Geometry check sheet. Reference: the model listing, model coordinates, mm. Give positions to 0.01 mm unless a question says otherwise; leave off trailing zeros. Order: outer loops, then holes, each group sorted by start corner. A loop starts at its lowest first (then second) coordinate and runs counter-clockwise, first axis right, second up. Notation, with made-up numbers: M 56.25,-34.5 L 88.25,-34.5 A31 ccw 88.25,-8.5 Z; hole C 69.25,71 d1. An arc over 180 degrees is marked long. Put each result on its own line as item: value. Start each with the question number.
Q1. Go/stop test with a flat-tipped pin: pin 1 (5.5 mm diameter, centred on x = -36, z = -4, fed in from -Y). Record where the tip stops, or that it passes through.
Q2. Section check C-C on y = 191. Record the cut outline in (x, z) (3 decimals), then the cut area to 3 significant figures.
Q3. Section check B-B on x = -40.5. Record the cut outline in (y, z) (3 decimals), then the cut area to 3 significant figures.
Q4. Section check D-D on z = -4.5. State how many separate pieces and enclosed holes the cut face has, then the cut area to 3 significant figures.
Q5. Material ranges on L1, parallel to X at y = -75.5, z = -6; L2, parallel to X at y = 268.5, z = 7.5; L3, parallel to Y at x = 256.5, z = -2, recorded low to high.
Q6. Section check A-A on x = 291. Record the cut outline in (y, z) (3 decimals).
```python
from build123d import *

# Parameters (mm, degrees)
SKETCH1_W           = 914.4
SKETCH1_H           = 914.4
BOSS_EXTRUDE1_DEPTH = 9.525
SKETCH2_W           = 184
SKETCH2_H           = 285
SKETCH2_W_2         = 300
SKETCH2_H_2         = 495
SKETCH2_W_3         = 469.9
SKETCH2_H_3         = 685.8
SKETCH2_H_4         = 177.8
CUT_EXTRUDE1_DEPTH  = 647.859012846
FILLET1_R           = 1


with BuildPart() as part:
    # Sketch1 → Boss-Extrude1 (new, symmetric)
    with BuildSketch(Plane.XY):
        Rectangle(SKETCH1_W, SKETCH1_H)
    extrude(amount=BOSS_EXTRUDE1_DEPTH, both=True)

    # Sketch2 → Cut-Extrude1 (cut, through all)
    with BuildSketch(Plane.XY.offset(9.525)):
        with Locations((292.1, 254)):
            Rectangle(SKETCH2_W, SKETCH2_H)
        with Locations((292.1, -177.8)):
            Rectangle(SKETCH2_W_2, SKETCH2_H_2)
        with Locations((-125.73, 101.6)):
            Rectangle(SKETCH2_W_3, SKETCH2_H_3)
        with Locations((-125.73, -368.3)):
            Rectangle(SKETCH2_W_3, SKETCH2_H_4)
    extrude(amount=-CUT_EXTRUDE1_DEPTH, mode=Mode.SUBTRACT)

    # Fillet1
    fillet1_edges = [part.edges().sort_by_distance(p)[0] for p in [
        (142.1, -425.3, 0),
        (142.1, 69.7, 0),
        (442.1, 69.7, 0),
        (442.1, -425.3, 0),
        (-360.68, -241.3, 0),
        (-360.68, 444.5, 0),
        (109.22, 444.5, 0),
        (109.22, -241.3, 0),
        (-360.68, -279.4, 0),
        (109.22, -279.4, 0),
        (200.1, 111.5, 0),
        (200.1, 396.5, 0),
        (384.1, 396.5, 0),
        (384.1, 111.5, 0),
    ]]
    fillet(fillet1_edges, radius=FILLET1_R)


solid = part.part
```
Results found:
1. pin 1: stops at y = -279.4
2. outline: M -457.2,-9.525 L -360.68,-9.525 L -360.68,9.525 L -457.2,9.525 Z; M 109.22,-9.525 L 200.1,-9.525 L 200.1,9.525 L 109.22,9.525 Z; M 384.1,-9.525 L 457.2,-9.525 L 457.2,9.525 L 384.1,9.525 Z
2. area: 4,960 mm^2
3. outline: M -279.4,-9.525 L -241.3,-9.525 L -241.3,9.525 L -279.4,9.525 Z; M 444.5,-9.525 L 457.2,-9.525 L 457.2,9.525 L 444.5,9.525 Z
3. area: 968 mm^2
4. separate pieces: 1
4. enclosed holes: 3
4. area: 229,000 mm^2
5. L1: x = -457.2 to -360.68, 109.22 to 142.1, 442.1 to 457.2
5. L2: x = -457.2 to -360.68, 109.22 to 200.1, 384.1 to 457.2
5. L3: y = -457.2 to -425.3, 69.7 to 111.5, 396.5 to 457.2
6. outline: M -457.2,-9.525 L -425.3,-9.525 L -425.3,9.525 L -457.2,9.525 Z; M 69.7,-9.525 L 111.5,-9.525 L 111.5,9.525 L 69.7,9.525 Z; M 396.5,-9.525 L 457.2,-9.525 L 457.2,9.525 L 396.5,9.525 Z
